Geometry check sheet. Reference: the model listing, model coordinates, mm. A direction names the side the tool comes from. Give positions to 0.01 mm unless a question says otherwise; leave off trailing zeros. Write each loop counter-clockwise with the first axis right and the second up, starting at its lowest first coordinate (ties: lowest second). Pieces come first, ordered by that corner, then holes. Notation, with made-up numbers: M 56,19 L 84,19 A7 cw 84,31 Z; hole C 10,26 d7. An arc over 180 degrees is marked long. Use one line per item in the form item = value. Start each with the question number.
```python
from build123d import *

# Parameters (mm, degrees)
SKETCH1_W                = 24
SKETCH1_H                = 34
BOSS_EXTRUDE1_DEPTH      = 11
CUT_EXTRUDE1_DEPTH       = 32.400636936
CUT_EXTRUDE2_DEPTH       = 38.69615365
SKETCH5_W                = 23
SKETCH5_H                = 33
CUT_EXTRUDE3_DEPTH       = 1.5
FILLET1_START            = -11.5
FILLET1_DEPTH            = 23
FILLET1_START_2          = -17
FILLET1_2_DEPTH          = 34
BOSS_EXTRUDE3_DEPTH      = 2
BOSS_EXTRUDE3_DEPTH_BACK = 2
SKETCH6_R                = 0.255
SKETCH8_R                = 1.203626853
BOSS_EXTRUDE4_DEPTH      = 0.001


with BuildPart() as part:
    # Sketch1 → Boss-Extrude1 (new body)
    with BuildSketch(Plane(origin=(0, 0, 0), x_dir=(1, 0, 0), z_dir=(0, 1, 0))):
        Rectangle(SKETCH1_W, SKETCH1_H)
    extrude(amount=BOSS_EXTRUDE1_DEPTH)

    # Sketch2 → Cut-Extrude1 (cut, through all)
    with BuildSketch(Plane(origin=(12, 0, 0), x_dir=(0, 0, -1), z_dir=(1, 0, 0))):
        Polygon((14.8, 1), (-14.8, 1), (-15, 0), (-15, -1), (15, -1), (15, 0), align=None)
    extrude(amount=-CUT_EXTRUDE1_DEPTH, mode=Mode.SUBTRACT)

    # Sketch3 → Cut-Extrude2 (cut, through all)
    with BuildSketch(Plane.XY.offset(17)):
        Polygon((9.8, 1), (-9.8, 1), (-10, 0), (-10, -1), (10, -1), (10, 0), align=None)
    extrude(amount=-CUT_EXTRUDE2_DEPTH, mode=Mode.SUBTRACT)

    # Sketch5 → Cut-Extrude3 (cut)
    with BuildSketch(Plane.XZ):
        Rectangle(SKETCH5_W, SKETCH5_H)
    extrude(amount=-CUT_EXTRUDE3_DEPTH, mode=Mode.SUBTRACT)

    # Fillet1: read off the stored shape, not the designer's step
    # Fillet1 outline → Fillet1 (add)
    with BuildSketch(Plane.YZ.offset(FILLET1_START)):
        with BuildLine():
            Line((1.5, 16.5), (1, 16.5))
            ThreePointArc((1, 16.5), (1.353553391, 16.353553391), (1.5, 16))
            Line((1.5, 16), (1.5, 16.5))
        make_face()
        with BuildLine():
            Line((1.5, -16.5), (1.5, -16))
            ThreePointArc((1.5, -16), (1.353553391, -16.353553391), (1, -16.5))
            Line((1, -16.5), (1.5, -16.5))
        make_face()
    extrude(amount=FILLET1_DEPTH)

    # Fillet1 2 outline → Fillet1 2 (add)
    with BuildSketch(Plane.XY.offset(FILLET1_START_2)):
        with BuildLine():
            Line((-11.5, 1.5), (-11.5, 1))
            ThreePointArc((-11.5, 1), (-11.353553391, 1.353553391), (-11, 1.5))
            Line((-11, 1.5), (-11.5, 1.5))
        make_face()
        with BuildLine():
            Line((11.5, 1.5), (11, 1.5))
            ThreePointArc((11, 1.5), (11.353553391, 1.353553391), (11.5, 1))
            Line((11.5, 1), (11.5, 1.5))
        make_face()
    extrude(amount=FILLET1_2_DEPTH)

    # Sketch6 → Boss-Extrude3 (add, two sides: drawn at the far end of the back side and taken through both)
    with BuildSketch(Plane.XZ.offset(-BOSS_EXTRUDE3_DEPTH_BACK)):
        with Locations(Location((0, 15.24, 0), (0, 0, 270))):
            Circle(SKETCH6_R)
        with Locations(Location((2.54, 15.24, 0), (0, 0, 270))):
            Circle(SKETCH6_R)
        with Locations(Location((5.08, 15.24, 0), (0, 0, 270))):
            Circle(SKETCH6_R)
        with Locations(Location((-5.08, 15.24, 0), (0, 0, 270))):
            Circle(SKETCH6_R)
        with Locations(Location((-2.54, 15.24, 0), (0, 0, 270))):
            Circle(SKETCH6_R)
        with Locations(Location((-2.54, -15.24, 0), (0, 0, 270))):
            Circle(SKETCH6_R)
        with Locations(Location((-5.08, -15.24, 0), (0, 0, 270))):
            Circle(SKETCH6_R)
        with Locations(Location((5.08, -15.24, 0), (0, 0, 270))):
            Circle(SKETCH6_R)
        with Locations(Location((2.54, -15.24, 0), (0, 0, 270))):
            Circle(SKETCH6_R)
        with Locations(Location((0, -15.24, 0), (0, 0, 270))):
            Circle(SKETCH6_R)
    extrude(amount=BOSS_EXTRUDE3_DEPTH + BOSS_EXTRUDE3_DEPTH_BACK)

    # Sketch8 → Boss-Extrude4 (add)
    with BuildSketch(Plane(origin=(0, 11, 0), x_dir=(1, 0, 0), z_dir=(0, 1, 0))):
        with Locations(Location((7.422365596, -11.514696897, 0), (0, 0, 270))):
            Circle(SKETCH8_R)
        with BuildLine():
            Line((4.437710207, -1.50424181), (3.234164607, -10.067913736))
            Line((3.234164607, -10.067913736), (4.862495803, -11.941094501))
            ThreePointArc((4.862495803, -11.941094501), (5.368748257, -11.200837396), (5.587567885, -10.331130491))
            Line((5.587567885, -10.331130491), (6.873174177, -1.183566406))
            Line((6.873174177, -1.183566406), (5.964953485, -0.043665222))
            Line((5.964953485, -0.043665222), (4.437710207, -1.50424181))
        make_face()
        with BuildLine():
            Line((5.877292712, 0.125030841), (7.205852999, 1.183566406))
            Line((7.205852999, 1.183566406), (8.491459291, 10.331130491))
            ThreePointArc((8.491459291, 10.331130491), (8.411955198, 11.093627172), (8.077597236, 11.783501683))
            Line((8.077597236, 11.783501683), (6.058508073, 10.028334252))
            Line((6.058508073, 10.028334252), (4.854667192, 1.462561294))
            Line((4.854667192, 1.462561294), (5.877292712, 0.125030841))
        make_face()
        with BuildLine():
            Line((6.10106331, 10.331130491), (7.952849968, 11.940864075))
            ThreePointArc((7.952849968, 11.940864075), (7.268624086, 12.470648357), (6.433742131, 12.698263303))
            Line((6.433742131, 12.698263303), (-2.864493083, 12.698263303))
            ThreePointArc((-2.864493083, 12.698263303), (-3.862201278, 12.569201297), (-4.732453708, 12.064484197))
            Line((-4.732453708, 12.064484197), (-3.197171904, 10.331130491))
            Line((-3.197171904, 10.331130491), (6.10106331, 10.331130491))
        make_face()
        Polygon((-4.815457018, -1.183566406), (4.482778196, -1.183566406), (5.720367413, 0), (4.815457018, 1.183566406), (-4.482778196, 1.183566406), (-5.844315597, 0), align=None)
        with BuildLine():
            Line((-5.975923975, 0.15139812), (-4.44022296, 1.486362645))
            Line((-4.44022296, 1.486362645), (-3.233869851, 10.07001103))
            Line((-3.233869851, 10.07001103), (-4.877500084, 11.925691561))
            ThreePointArc((-4.877500084, 11.925691561), (-5.373142616, 11.19102491), (-5.587567885, 10.331130491))
            Line((-5.587567885, 10.331130491), (-6.873174177, 1.183566406))
            Line((-6.873174177, 1.183566406), (-5.975923975, 0.15139812))
        make_face()
        with BuildLine():
            Line((-5.995713717, -0.131608377), (-7.205852999, -1.183566406))
            Line((-7.205852999, -1.183566406), (-8.491459291, -10.331130491))
            ThreePointArc((-8.491459291, -10.331130491), (-8.411955198, -11.093627172), (-8.077597236, -11.783501683))
            Line((-8.077597236, -11.783501683), (-6.058508073, -10.028334252))
            Line((-6.058508073, -10.028334252), (-4.85244972, -1.446783161))
            Line((-4.85244972, -1.446783161), (-5.995713717, -0.131608377))
        make_face()
        with BuildLine():
            Line((-6.10106331, -10.331130491), (-7.952849968, -11.940864075))
            ThreePointArc((-7.952849968, -11.940864075), (-7.268624086, -12.470648357), (-6.433742131, -12.698263303))
            Line((-6.433742131, -12.698263303), (2.864493083, -12.698263303))
            ThreePointArc((2.864493083, -12.698263303), (3.852009379, -12.572635363), (4.716279741, -12.078664154))
            Line((4.716279741, -12.078664154), (3.197171904, -10.331130491))
            Line((3.197171904, -10.331130491), (-6.10106331, -10.331130491))
        make_face()
    extrude(amount=BOSS_EXTRUDE4_DEPTH)


solid = part.part
```
(1) Thickness scan on probe 1 along Y at (x, z) = (-4.5, 10). Record the ranges inside material, lowest first. Write a range as [from, to].
(2) Sectioned sample at A-A, the plane y = -0.75. State how many separate pieces and enclosed holes the cut face has, plus the area to 3 significant figures.
(3) Sectioned sample at B-B, the plane z = -14. Record the boundary of the cut face in (x, y).
(4) Sectioned sample at C-C, the plane x = -10.5. Record the boundary of the cut face in (y, z), plus the area to 3 significant figures.
(5) Draft check along Z on faces 1 (the flat face through (-10.7, 0.5, -16.5)), 2 (the flat face through (-11.5, 0, -16.7)). Enter one of: released by +Z, released by -Z, zero draft, split by the parting line, or undercut.
(6) Tool access check on faces 3 (the flat face through (-11.5, 0.5, -15.7)), 4 (the flat face through (0, 11, -4)). Record the directions out of +Z, -Z, +X, -X, +Y, -Y that give a thin tool (end or side, any length) a straight path to the whole face; none if there is none.
(7) Depth check by flat-ended pin: pin 1 (1.5 mm diameter, centred on x = -2.5, z = 7, fed in from -Y); pin 2 (2 mm diameter, centred on x = 11.5, z = 16, fed in from -Y). Enter the tip coordinate at first touch or a pass-through.
Numbers:
q1.probe_1 = [1.5, 11]
q2.separate_pieces = 10
q2.enclosed_holes = 0
q2.area = 2.04 mm2
q3.outline = M -12,1 L -11.5,1 A0.5 cw -11,1.5 L 11,1.5 A0.5 cw 11.5,1 L 12,1 L 12,11 L -12,11 Z
q4.outline = M 0,-17 L 11,-17 L 11,17 L 0,17 L 0,16.5 L 1,16.5 A0.5 cw 1.5,16 L 1.5,-16 A0.5 cw 1,-16.5 L 0,-16.5 Z
q4.area = 325 mm2
q5.face_1 = undercut
q5.face_2 = zero draft
q6.face_3 = -Y
q6.face_4 = +Z, -Z, +X, -X, +Y
q7.pin_1 = 1.5
q7.pin_2 = 0
